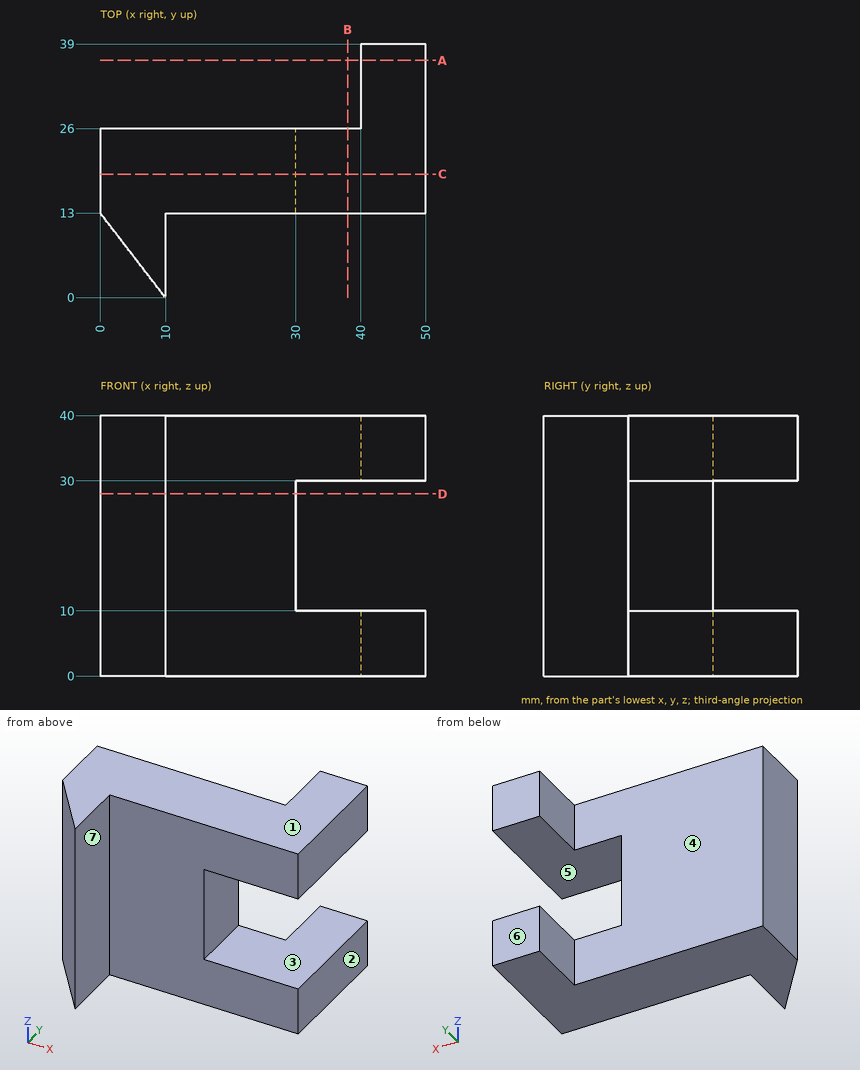
Check sheet for the drawn part. Datum: minimum x, y, z corner. Units: mm. A direction names the side the tool comes from. Give positions to 0.01 mm unless a question says otherwise; leave off trailing zeros. Order: outer loops, then holes, each group sorted by start corner. A loop starts at its lowest first (then second) coordinate and runs counter-clockwise, first axis right, second up.
1. Depth check by flat-ended pin: pin 1 (1.5 mm diameter, centred on x = 9, z = 33.5, fed in from -Y) (3 decimals); pin 2 (6 mm diameter, centred on y = 6, z = 30.5, fed in from -X); pin 3 (3 mm diameter, centred on x = 5.5, z = 10, fed in from -Y). Enter the tip coordinate at first touch or a pass-through.
Completed:
pin 1: stops at y = 0.325
pin 2: stops at x = 3.08
pin 3: stops at y = 3.9
2. Access from +Z, -Z, +X, -X, +Y, -Y to the whole of each face (thin tool, end or side, straight path). Record for the marked faces 4, 5, 6 and 7.
Completed:
face 4: +Z, -Z, -X, +Y
face 5: +X, +Y, -Y
face 6: +Z, -Z, +X, -X, +Y
face 7: +Z, -Z, +X, -Y
3. Sectioned sample at A-A (y = 36.5). Record the boundary of the cut face in (x, z), then the cut area to 3 significant figures.
Completed:
outline: (40, 0) - (50, 0) - (50, 10) - (40, 10) - close; (40, 30) - (50, 30) - (50, 40) - (40, 40) - close
area: 200 mm2
4. Scan lines: line 1 (Z direction, x = 36, y = 25.5); line 2 (Y direction, x = 33, z = 37.5); line 3 (Y direction, x = 42.5, z = 5.5). Record each from-to range of solid material in increasing order.
Completed:
line 1: z = 0 to 10, 30 to 40
line 2: y = 13 to 26
line 3: y = 13 to 39
5. Draft check along Z on the marked faces 1, 2 and 3. Enter one of: pulls with the +Z half, pulls with the -Z half, needs draft (parallel to the pull), parting line crosses it, or undercut.
Completed:
face 1: pulls with the +Z half
face 2: needs draft
face 3: undercut
6. Sectioned sample at C-C (y = 19). Record the boundary of the cut face in (x, z), then the cut area to 3 significant figures.
Completed:
outline: (0, 0) - (50, 0) - (50, 10) - (30, 10) - (30, 30) - (50, 30) - (50, 40) - (0, 40) - close
area: 1,600 mm2
7. Sectioned sample at D-D (z = 28). Record the boundary of the cut face in (x, y).
Completed:
outline: (0, 13) - (10, 0) - (10, 13) - (30, 13) - (30, 26) - (0, 26) - close
8. Sectioned sample at B-B (x = 38). Record the boundary of the cut face in (y, z), then the cut area to 3 significant figures.
Completed:
outline: (13, 0) - (26, 0) - (26, 10) - (13, 10) - close; (13, 30) - (26, 30) - (26, 40) - (13, 40) - close
area: 260 mm2
